Build history of the part. All positions in model axes, mm. A direction names the side the tool comes from. Coordinates: 2 decimals unless noted, no trailing zeros. Order: outer loops, then holes, each group sorted by start corner. A loop starts at its lowest first (then second) coordinate and runs counter-clockwise, first axis right, second up. Notation, with made-up numbers: (-24.75, 42.25) - (-12.75, 42.25) arc R29 cw to (-12.75, 66.25) - close; hole circle Ø9 at (84, -4). An arc over 180 degrees is marked (long way). Return JSON: item names as keys, results as strings.
from build123d import *

# Parameters (mm, degrees)
POCKET002_DEPTH = 7.5
PAD001_DEPTH    = 2


with BuildPart() as part:
    # Sketch004 → Revolution001 (revolve)
    with BuildSketch(Plane.YZ):
        Polygon((0, -22), (27.72376, -22), (27.72376, -14.5), (29.22376, -14.5), (29.97376, -16), (29.22376, -17.5), (29.22376, -24), (0, -24), align=None)
    revolve(axis=Axis((0, 0, 0), (0, 0, 1)))

    # Sketch005 (on Face3 of Revolution001) → Pocket002 (cut)
    with BuildSketch(Plane(origin=(0, 0, -14.5), x_dir=(0, -1, 0), z_dir=(0, 0, 1))):
        Polygon((-12.5, 31.22376), (12.5, 31.22376), (12.5, 21.650635), (20.790569, 26.437197), (33.290569, 4.786562), (25, 0), (33.290569, -4.786562), (20.790569, -26.437197), (12.5, -21.650635), (12.5, -31.22376), (-12.5, -31.22376), (-12.5, -21.650635), (-20.790569, -26.437197), (-33.290569, -4.786562), (-25, 0), (-33.290569, 4.786562), (-20.790569, 26.437197), (-12.5, 21.650635), align=None)
    extrude(amount=-POCKET002_DEPTH, mode=Mode.SUBTRACT)

    # Sketch006 (on Face39 of Pocket002) → Pad001 (join)
    with BuildSketch(Plane.YX.offset(24)):
        with BuildLine():
            ThreePointArc((5.5, 32.258246), (0, 32.72376), (-5.5, 32.258246))
            Line((-5.5, 32.258246), (-5.5, 0))
            Line((5.5, 0), (-5.5, 0))
            Line((5.5, 32.258246), (5.5, 0))
        make_face()
    extrude(amount=-PAD001_DEPTH)


solid = part.part
1. Cut at B-B on y = 0. Give the cut face in (x, z).
Check values:
{"outline": "(-29.22, -24) - (32.72, -24) - (32.72, -22) - (-29.22, -22) - close"}
2. Probe L1, parallel to Z at x = 8.5, y = 0.5; L2, parallel to Y at x = 23.5, z = -21.75; L3, parallel to X at y = -13, z = -21. List the from-to ranges inside material, lowest first.
Check values:
{"L1": "-24 to -22", "L2": "-15.7 to -14.71, 14.71 to 15.7", "L3": "-26.17 to -24.49, 24.49 to 26.17"}
3. Cut at C-C on x = 12.5. Give the cut face in (y, z).
Check values:
{"outline": "(-26.42, -24) - (26.42, -24) - (26.42, -22) - (-26.42, -22) - close"}
4. Tool access for faces 4 (the flat face through (2.042, -28.537, -18.197)), 5 (the flat face through (31, -5.5, -23)), 6 (the flat face through (-2.024, -28.506, -18.197)): list every direction of +Z, -Z, +X, -X, +Y, -Y with a clear straight run to the whole face (end or side of a thin tool).
Check values:
{"face 4": "+Z, +X", "face 5": "+Z, -Z, +X, -Y", "face 6": "+Z, -X"}
5. Cut at A-A on x = 0. Give the cut face in (y, z), plus the area to 3 significant figures.
Check values:
{"outline": "(-29.97, -16) - (-29.22, -17.5) - (-29.22, -24) - (29.22, -24) - (29.22, -17.5) - (29.97, -16) - (29.22, -14.5) - (27.72, -14.5) - (27.72, -22) - (-27.72, -22) - (-27.72, -14.5) - (-29.22, -14.5) - close", "area": "142 mm²"}
6. Mould opens along X. For faces 1 (the flat face through (-25, -14, -14.5)), 2 (the conical face through (25.657, 14.768, -15.261)), 3 (the cylindrical face through (-24.02, -13.84, -18.2)) say: pulls with the +X half, pulls with the -X half, needs draft (parallel to the pull), parting line crosses it, or undercut.
Check values:
{"face 1": "needs draft", "face 2": "pulls with the +X half", "face 3": "undercut"}
7. Drop flat-ended pins along their axis: pin 1 (2.5 mm diameter, centred on x = 26.5, z = -18, fed in from +Y); pin 2 (0.7 mm diameter, centred on x = 26, z = -16.5, fed in from -Y); pin 3 (1.2 mm diameter, centred on x = -26, z = -19, fed in from +Y). Give the stop position or say it passes through.
Check values:
{"pin 1": "y = 14.71", "pin 2": "y = -15.11", "pin 3": "y = 14.45"}
